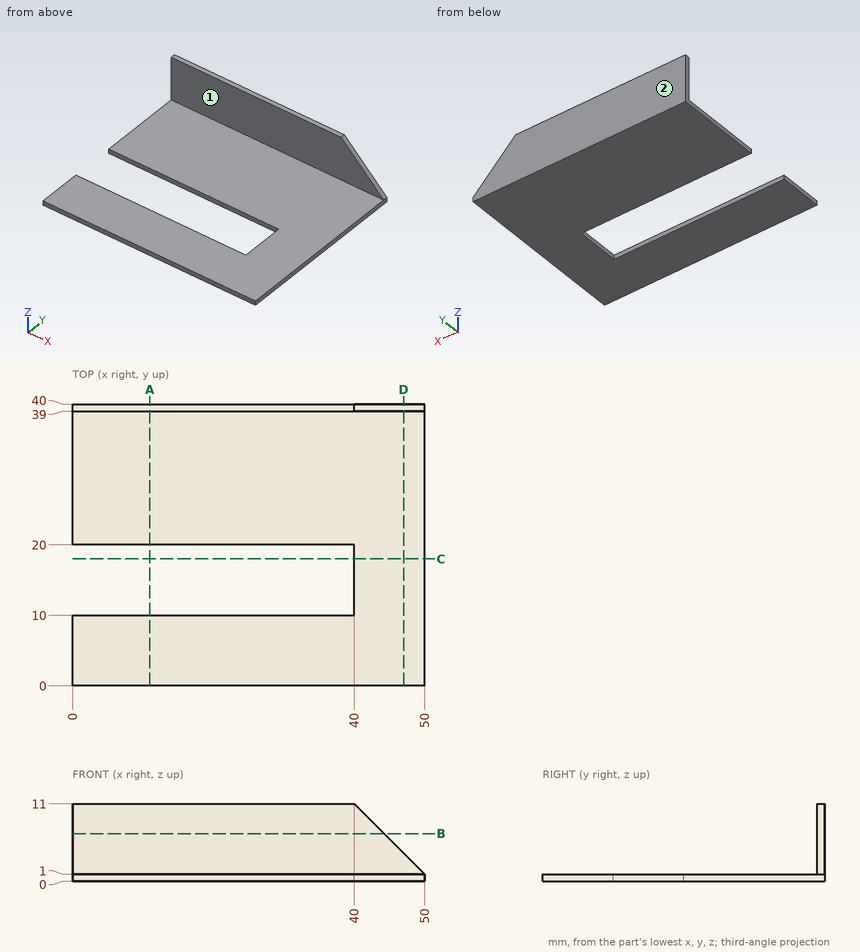
The figure shows three views and two pictorial views of one solid part (mm, origin at its lowest corner). Answer the questions. A direction names the side the tool comes from. Round coordinates to 2 decimals unless told otherwise and drop trailing zeros. Loops run counter-clockwise (first coordinate to the right, second up) from the corner with the lowest first, then second, coordinate; pieces in that order, holes last. Notation, with made-up numbers: (46.5, 67.25) - (83.5, 67.25) arc R22 cw to (83.5, 95.25) - close; hole circle Ø4 at (53, -3.75). An arc over 180 degrees is marked (long way). One line per question, with ' | ' between items. Start each with the question number.
Q1. Section B-B on z = 6.75 is taken. Give the vertices of the cut face in (x, y).
Q2. Section A-A on x = 11 is taken. Give the vertices of the cut face in (y, z), plus the area to 3 significant figures.
Q3. Find the intervals of material crossed by L1, parallel to Y at x = 35.5, z = 6.5; L2, parallel to Z at x = 48.5, y = 16.5, in increasing order.
Q4. For the marked faces 1 and 2, determine the directions among +Z, -Z, +X, -X, +Y, -Y from which every point of the face is accessible in a straight line to the end or side of a thin tool.
Q5. Section D-D on x = 47 is taken. Give the vertices of the cut face in (y, z), plus the area to 3 significant figures.
Q6. Flat-ended cylindrical pins translate along their axes: pin 1 (5 mm diameter, centred on x = 17.5, y = 4.5, fed in from +Z); pin 2 (4 mm diameter, centred on y = 36, z = 5.5, fed in from +X); pin 3 (5 mm diameter, centred on x = 17.5, z = 7.5, fed in from -Y). Find the tip coordinate at first contact, or state that the pin passes through.
Q7. Section C-C on y = 18 is taken. Give the vertices of the cut face in (x, z), plus the area to 3 significant figures.
Established:
1) outline: (0, 39) - (44.25, 39) - (44.25, 40) - (0, 40) - close
2) outline: (0, 0) - (10, 0) - (10, 1) - (0, 1) - close; (20, 0) - (40, 0) - (40, 11) - (39, 11) - (39, 1) - (20, 1) - close | area: 40.0 mm²
3) L1: 39 to 40 | L2: 0 to 1
4) face 1: +Z, +X, -X, -Y | face 2: +Z, -Z, +X, -X, +Y
5) outline: (0, 0) - (40, 0) - (40, 4) - (39, 4) - (39, 1) - (0, 1) - close | area: 43.0 mm²
6) pin 1: z = 1 | pin 2: through | pin 3: y = 39
7) outline: (40, 0) - (50, 0) - (50, 1) - (40, 1) - close | area: 10.0 mm²
